```python
from build123d import *

# Parameters (mm, degrees)
BOSS_EXTRUDE1_DEPTH = 10
SKETCH2_R           = 2.75
CUT_EXTRUDE1_DEPTH  = 29.08914381
SKETCH3_R           = 2.75
CUT_EXTRUDE2_DEPTH  = 26.377155081
RIB7_REACH          = 35
SKETCH5_WALL_W      = 87.209372712
SKETCH5_WALL_H      = 3
RIB8_REACH          = 35
SKETCH6_WALL_W      = 87.209372712
SKETCH6_WALL_H      = 3
FILLET1_R           = 1
FILLET2_R           = 1


with BuildPart() as part:
    # Sketch1 → Boss-Extrude1 (new, symmetric)
    with BuildSketch(Plane.XY):
        Polygon((0, 0), (0, 12), (-15, 12), (-15, 17), (5, 17), (5, 5), (20, 5), (20, 0), align=None)
    extrude(amount=BOSS_EXTRUDE1_DEPTH, both=True)

    # Sketch2 → Cut-Extrude1 (cut, through all)
    with BuildSketch(Plane(origin=(0, 17, 0), x_dir=(1, 0, 0), z_dir=(0, 1, 0))):
        with Locations(Location((-8, 0, 0), (0, 0, 270))):
            Circle(SKETCH2_R)
    extrude(amount=-CUT_EXTRUDE1_DEPTH, mode=Mode.SUBTRACT)

    # Sketch3 → Cut-Extrude2 (cut, through all)
    with BuildSketch(Plane(origin=(0, 5, 0), x_dir=(1, 0, 0), z_dir=(0, 1, 0))):
        with Locations(Location((13, 0, 0), (0, 0, 180))):
            Circle(SKETCH3_R)
    extrude(amount=-CUT_EXTRUDE2_DEPTH, mode=Mode.SUBTRACT)

    # Sketch5 wall → Rib7 (add, up to next)
    with BuildSketch(Plane(origin=(12.5, 11, -10), x_dir=(-0.780868809443, 0.624695047554, 0), z_dir=(0.624695047554, 0.780868809443, 0)), mode=Mode.PRIVATE) as rib7_sk1:
        with Locations((0, 1.5)):
            Rectangle(SKETCH5_WALL_W, SKETCH5_WALL_H)
    rib7_tool1 = extrude(rib7_sk1.sketch, amount=-RIB7_REACH, mode=Mode.PRIVATE) - part.part
    rib7 = rib7_tool1.solids().sort_by_distance((12.5, 11, -10))[0]
    add(rib7)

    # Sketch6 wall → Rib8 (add, up to next)
    with BuildSketch(Plane(origin=(-7.5, 6, -10), x_dir=(0.780868809443, -0.624695047554, 0), z_dir=(-0.624695047554, -0.780868809443, 0)), mode=Mode.PRIVATE) as rib8_sk1:
        with Locations((0, 1.5)):
            Rectangle(SKETCH6_WALL_W, SKETCH6_WALL_H)
    rib8_tool1 = extrude(rib8_sk1.sketch, amount=-RIB8_REACH, mode=Mode.PRIVATE) - part.part
    rib8 = rib8_tool1.solids().sort_by_distance((-7.5, 6, -10))[0]
    add(rib8)

    # Mirror1: Rib7, Rib8 across plane
    add(rib7.mirror(Plane.XY))
    add(rib8.mirror(Plane.XY))

    # Fillet1
    fillet1_edges = [part.edges().sort_by_distance(p)[0] for p in [
        (0, 12, 0),
        (-7.5, 12, 7),
        (0, 6, 7),
        (5, 11, -7),
        (12.5, 5, -7),
        (0, 6, -7),
        (-7.5, 12, -7),
        (5, 5, 0),
        (12.5, 5, 7),
        (5, 11, 7),
    ]]
    fillet(fillet1_edges, radius=FILLET1_R)

    # Fillet2
    fillet2_edges = [part.edges().sort_by_distance(p)[0] for p in [
        (20, 2.5, -10),
        (-15, 14.5, 10),
        (20, 2.5, 10),
        (-15, 14.5, -10),
    ]]
    fillet(fillet2_edges, radius=FILLET2_R)


solid = part.part
```
CAD build for the part. Positions are in the model's coordinates, mm. A direction names the side the tool comes from. Round coordinates to 2 decimals unless told otherwise and drop trailing zeros. Order: outer loops, then holes, each group sorted by start corner. A loop starts at its lowest first (then second) coordinate and runs counter-clockwise, first axis right, second up.
Q1. Slice it at D-D (y = 8). Write the cut outline in (x, z), and give its area (3 significant figures).
Q2. Slice it at C-C (x = 13). Write the cut outline in (y, z).
Q3. Wall check: L1, parallel to Z at x = 13, y = 3.4; L2, parallel to Z at x = -6, y = 8.75; L3, parallel to X at y = 13.7, z = 0. Give the ranges that are in metal, low to high.
Q4. Slice it at B-B (z = 0). Write the cut outline in (x, y).
Q5. Slice it at A-A (y = 3). Write the cut outline in (x, z), and give its area (3 significant figures).
Q6. Drop flat-ended pins along their axis: pin 1 (5 mm diameter, centred on y = 12.5, z = 5.5, fed in from +X) (3 decimals); pin 2 (9 mm diameter, centred on y = 5.5, z = -0.5, fed in from -X); pin 3 (5 mm diameter, centred on x = 13, z = 0, fed in from -Y); pin 4 (6 mm diameter, centred on x = 14.5, z = 0.5, fed in from +Y). Give the stop position or say it passes through.
Q7. Which spindle directions (+Z, -Z, +X, -X, +Y, -Y) get a long thin tool onto all of the face, cutting with end or side? Do faces 5 (the cylindrical face through (5.285, 5.301, -0.084)), 6 (the flat face through (-8, 12, 3)), 7 (the cylindrical face through (-14.699, 14.141, 9.715)). Say none if no direction does.
Q8. Two-plate mould, pull along Z, no slides. Class faces 1 (the cylindrical face through (19.699, 2.859, -9.715)), 2 (the cylindrical face through (12.902, 5.285, 6.699)), 3 (the cylindrical face through (19.715, 2.859, 9.699)), 4 (the flat face through (12.605, 10.916, 8.416)): pulls with the +Z half, pulls with the -Z half, needs draft (parallel to the pull), parting line crosses it, or undercut.
Results below:
1. outline: (-10, -10) - (16.25, -10) - (16.25, -7) - (6, -7) arc R1 cw to (5, -6) - (5, 6) arc R1 cw to (6, 7) - (16.25, 7) - (16.25, 10) - (-10, 10) - (-10, 7) - (-1, 7) arc R1 cw to (0, 6) - (0, -6) arc R1 cw to (-1, -7) - (-10, -7) - close
1. area: 228 mm2
2. outline: (0, -10) - (10.6, -10) - (10.6, -7) - (6, -7) arc R1 cw to (5, -6) - (5, -2.75) - (0, -2.75) - close; (0, 2.75) - (5, 2.75) - (5, 6) arc R1 cw to (6, 7) - (10.6, 7) - (10.6, 10) - (0, 10) - close
3. L1: z = -10 to -2.75, 2.75 to 10
3. L2: z = -10 to -7, 7 to 10
3. L3: x = -15 to -10.75, -5.25 to 5
4. outline: (-15, 12) - (-10.75, 12) - (-10.75, 17) - (-15, 17) - close; (-5.25, 12) - (-1, 12) arc R1 cw to (0, 11) - (0, 0) - (10.25, 0) - (10.25, 5) - (6, 5) arc R1 cw to (5, 6) - (5, 17) - (-5.25, 17) - close; (15.75, 0) - (20, 0) - (20, 5) - (15.75, 5) - close
5. outline: (-3.75, -10) - (19, -10) arc R1 ccw to (20, -9) - (20, 9) arc R1 ccw to (19, 10) - (-3.75, 10) - (-3.75, 7) - (-1, 7) arc R1 cw to (0, 6) - (0, -6) arc R1 cw to (-1, -7) - (-3.75, -7) - close; hole circle Ø5.5 at (13, 0)
5. area: 399 mm2
6. pin 1: stops at x = 13.125
6. pin 2: stops at x = 0
6. pin 3: passes through
6. pin 4: stops at y = 5
7. face 5: +X, +Y
7. face 6: -X, -Y
7. face 7: +Z, -X, +Y, -Y
8. face 1: pulls with the -Z half
8. face 2: undercut
8. face 3: pulls with the +Z half
8. face 4: needs draft
